Here's how the part is built. I have some questions about the finished solid (model axes, mm). A direction names the side the tool comes from. Round coordinates to 2 decimals unless told otherwise and drop trailing zeros. Order: outer loops, then holes, each group sorted by start corner. A loop starts at its lowest first (then second) coordinate and runs counter-clockwise, first axis right, second up. Notation, with made-up numbers: (28, -4) -> (55, -4) arc R17 ccw to (55, 22) -> close; hole circle Ø11 at (24, 51). An arc over 180 degrees is marked (long way). Use a Markdown table: item, result. Add a question column.
(1) Thinking about a two-plate mould opening in X: for faces 3 (the face through (-60.327, 0.042, 74.127)), 4 (the face through (-1, -3, -1)), 5 (the face through (0.1, 0.04, -82.55)), 6 (the face through (42.98, 0.04, -87.58)), which applies, pulls with the +X half, pulls with the -X half, needs draft (parallel to the pull), parting line crosses it, or undercut?
(2) I want a section at A-A, the plane y = -0.5. Give the number of separate pieces and of enclosed holes in the cut face, then the cut area to 3 significant figures.
(3) If I drill on probe 1 along Z at (x, y) = (0, -1.25); probe 2 along Z at (x, y) = (-51, -2.5); probe 3 along Z at (x, y) = (-18.5, -0.5), over which ranges is the centre line in solid material (lowest first)?
(4) I want a section at B-B, the plane z = 49.5. Please give me the cut outline in (x, y), then the cut area to 3 significant figures.
(5) I want a section at C-C, the plane x = -35.5. Please give me the cut outline in (y, z).
(6) On a 3-axis mill with a long thin cutter (end or side, diameter ignored), from which of +Z, -Z, +X, -X, +Y, -Y can I reach the whole of each face in a straight line? I mean faces 1 (the face through (-60.3, 0.04, -74.28)), 2 (the face through (16.757, 0.042, 84.451)). Say none if no direction works.
(7) I'm going to push a flat-ended pin straight in: P1, Ø2, axis at x = 75.61, z = 24.57, coming from the -Y side. Where does the tip first touch, or does it pass through?
from build123d import *

# Parameters (mm, degrees)
SKETCH1_R            = 2.75
BOSS_EXTRUDE1_DEPTH  = 3
M3_CLEARANCE_HOLE1_D = 3.4
FILLET2_R            = 10


with BuildPart() as part:
    # Sketch1 → Boss-Extrude1 (new, symmetric)
    with BuildSketch(Plane(origin=(0, 0, 0), x_dir=(1, 0, 0), z_dir=(0, 1, 0))):
        with BuildLine():
            Line((-58.614111744, 67.959966353), (-53.914904373, 62.511483636))
            ThreePointArc((-53.914904373, 62.511483636), (-82.55, 0), (-53.914904373, -62.511483636))
            Line((-53.914904373, -62.511483636), (-58.614111744, -67.959966353))
            ThreePointArc((-58.614111744, -67.959966353), (-60.384815089, -73.721869234), (-57.34308106, -78.925980035))
            ThreePointArc((-57.34308106, -78.925980035), (-42.766558206, -87.684438581), (-26.890595122, -93.77864983))
            ThreePointArc((-26.890595122, -93.77864983), (-20.917021387, -92.971598421), (-17.46673379, -88.028883515))
            Line((-17.46673379, -88.028883515), (-16.066391761, -80.971436666))
            ThreePointArc((-16.066391761, -80.971436666), (0, -82.55), (16.066391761, -80.971436666))
            Line((16.066391761, -80.971436666), (17.46673379, -88.028883515))
            ThreePointArc((17.46673379, -88.028883515), (20.917021387, -92.971598421), (26.890595122, -93.77864983))
            ThreePointArc((26.890595122, -93.77864983), (42.766558206, -87.684438581), (57.34308106, -78.925980035))
            ThreePointArc((57.34308106, -78.925980035), (60.384815089, -73.721869234), (58.614111744, -67.959966353))
            Line((58.614111744, -67.959966353), (53.914904373, -62.511483636))
            ThreePointArc((53.914904373, -62.511483636), (82.55, 0), (53.914904373, 62.511483636))
            Line((53.914904373, 62.511483636), (58.614111744, 67.959966353))
            ThreePointArc((58.614111744, 67.959966353), (60.384815089, 73.721869234), (57.34308106, 78.925980035))
            ThreePointArc((57.34308106, 78.925980035), (42.766558206, 87.684438581), (26.890595122, 93.77864983))
            ThreePointArc((26.890595122, 93.77864983), (20.917021387, 92.971598421), (17.46673379, 88.028883515))
            Line((17.46673379, 88.028883515), (16.066391761, 80.971436666))
            ThreePointArc((16.066391761, 80.971436666), (0, 82.55), (-16.066391761, 80.971436666))
            Line((-16.066391761, 80.971436666), (-17.46673379, 88.028883515))
            ThreePointArc((-17.46673379, 88.028883515), (-20.917021387, 92.971598421), (-26.890595122, 93.77864983))
            ThreePointArc((-26.890595122, 93.77864983), (-42.766558206, 87.684438581), (-57.34308106, 78.925980035))
            ThreePointArc((-57.34308106, 78.925980035), (-60.384815089, 73.721869234), (-58.614111744, 67.959966353))
        make_face()
        with Locations(Location((52.934691668, -72.858352577, 0), (0, 0, 270))):
            Circle(SKETCH1_R, mode=Mode.SUBTRACT)
        with Locations(Location((52.934691668, 72.858352577, 0), (0, 0, 90))):
            Circle(SKETCH1_R, mode=Mode.SUBTRACT)
        with Locations(Location((-52.934691668, -72.858352577, 0), (0, 0, 90))):
            Circle(SKETCH1_R, mode=Mode.SUBTRACT)
        with Locations(Location((-52.934691668, 72.858352577, 0), (0, 0, 270))):
            Circle(SKETCH1_R, mode=Mode.SUBTRACT)
    extrude(amount=BOSS_EXTRUDE1_DEPTH, both=True)

    # M3 Clearance Hole1 (through all)
    with Locations(Plane(origin=(0, 3, 0), x_dir=(1, 0, 0), z_dir=(0, 1, 0))):
        with Locations((0, 79.5), (46.728927557, 64.316851053), (75.608993045, 24.566851053), (75.608993045, -24.566851053), (46.728927557, -64.316851053), (0, -79.5), (-46.728927557, -64.316851053), (-75.608993045, -24.566851053), (-75.608993045, 24.566851053), (-46.728927557, 64.316851053)):
            Hole(M3_CLEARANCE_HOLE1_D / 2)

    # Fillet2
    fillet2_edges = [part.edges().sort_by_distance(p)[0] for p in [
        (-53.914904373, 0, 62.511483636),
        (-53.914904373, 0, -62.511483636),
        (-16.066391761, 0, 80.971436666),
        (53.914904373, 0, 62.511483636),
        (53.914904373, 0, -62.511483636),
        (16.066391761, 0, -80.971436666),
        (-16.066391761, 0, -80.971436666),
    ]]
    fillet(fillet2_edges, radius=FILLET2_R)


solid = part.part
Taken from the geometry:
| question | item | result |
|---|---|---|
| 1 | face 3 | pulls with the -X half |
| 1 | face 4 | needs draft |
| 1 | face 5 | undercut |
| 1 | face 6 | pulls with the +X half |
| 2 | separate pieces | 1 |
| 2 | enclosed holes | 14 |
| 2 | area | 24,000 mm2 |
| 3 | probe 1 | z = -82.55 to -81.2, -77.8 to 77.8, 81.2 to 82.55 |
| 3 | probe 2 | z = -83.17 to -74.81, -70.9 to 70.9, 74.81 to 83.17 |
| 3 | probe 3 | z = -90.6 to 90.6 |
| 4 | outline | (-66.06, -3) -> (66.06, -3) -> (66.06, 3) -> (-66.06, 3) -> close |
| 4 | area | 793 mm2 |
| 5 | outline | (-3, -90.87) -> (3, -90.87) -> (3, 90.87) -> (-3, 90.87) -> close |
| 6 | face 1 | -X, +Y, -Y |
| 6 | face 2 | +Z, +Y, -Y |
| 7 | P1 | passes through |
